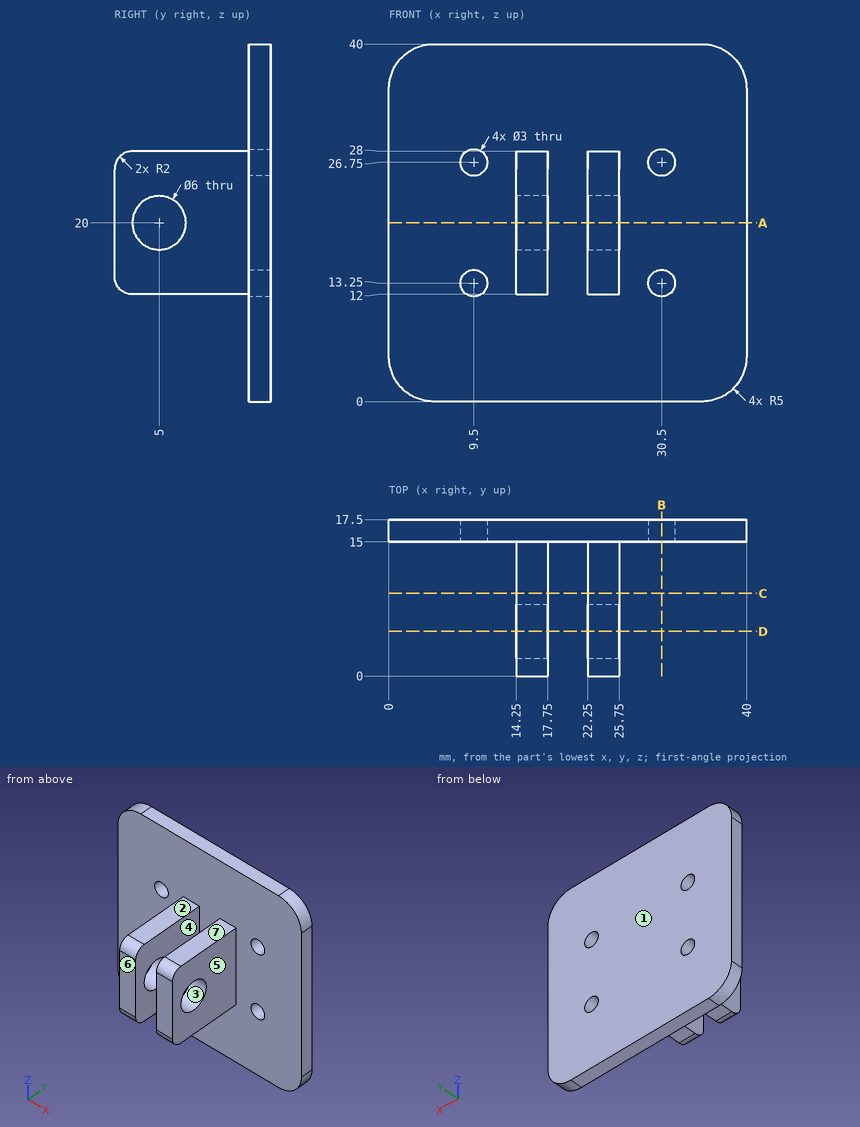
The drawing under review shows one solid part. Ordinate dimensions are in mm from its lowest x, y, z. A direction names the side the tool comes from. Coordinates: 2 decimals unless noted, no trailing zeros. Write each loop counter-clockwise with the first axis right and the second up, starting at its lowest first coordinate (ties: lowest second). Pieces come first, ordered by that corner, then holes.
1) Mouldability with a two-part tool opening along Y and no side actions: class the marked faces 1, 2 and 3 as +Y half, -Y half, draft (parallel to the pull), parting line (faces both ways), or undercut.
2) Add section D-D (y = 5). Write out the cut boundary in (x, z).
3) Add section B-B (x = 30.5). Write out the cut boundary in (y, z).
4) Add section C-C (y = 9.25). Write out the cut boundary in (x, z).
5) Machinability: for the marked faces 4, 5, 6 and 7, which of the approach directions +Z, -Z, +X, -X, +Y, -Y give a long, thin tool a straight path to every point of the face, cutting with its end or side? Answer none if there is none.
6) Add section A-A (z = 20). Write out the cut boundary in (x, y), plus the area to 3 significant figures.
7) To check wall thickness, follow L1, parallel to X at y = 16.25, z = 13.25; L2, parallel to X at y = 9, z = 17.5; L3, parallel to Y at x = 15, z = 20. State the ranges of each line that lie inside material, in increasing order.
8) Insertion check: pin 1 (2.5 mm diameter, centred on x = 9.5, z = 13.25, fed in from +Y); pin 2 (3 mm diameter, centred on y = 9, z = 17, fed in from +X); pin 3 (1.8 mm diameter, centred on x = 23.5, y = 9.5, fed in from +Z); pin 4 (12 mm diameter, centred on x = 13.5, z = 17, fed in from -Y). Each pin has a flat end and moves straight along its axis. Give the tip position at first contact, or say it passes through.
Check result:
1. face 1: +Y half
1. face 2: draft
1. face 3: undercut
2. outline: (14.25, 12) - (17.75, 12) - (17.75, 17) - (14.25, 17) - close; (14.25, 23) - (17.75, 23) - (17.75, 28) - (14.25, 28) - close; (22.25, 12) - (25.75, 12) - (25.75, 17) - (22.25, 17) - close; (22.25, 23) - (25.75, 23) - (25.75, 28) - (22.25, 28) - close
3. outline: (15, 0) - (17.5, 0) - (17.5, 11.75) - (15, 11.75) - close; (15, 14.75) - (17.5, 14.75) - (17.5, 25.25) - (15, 25.25) - close; (15, 28.25) - (17.5, 28.25) - (17.5, 40) - (15, 40) - close
4. outline: (14.25, 12) - (17.75, 12) - (17.75, 28) - (14.25, 28) - close; (22.25, 12) - (25.75, 12) - (25.75, 28) - (22.25, 28) - close
5. face 4: +Z, -Z, -Y
5. face 5: +Z, -Z, +X, -Y
5. face 6: +Z, -Z, +X, -X, -Y
5. face 7: +Z, +X, -X, -Y
6. outline: (0, 15) - (14.25, 15) - (14.25, 8) - (17.75, 8) - (17.75, 15) - (22.25, 15) - (22.25, 8) - (25.75, 8) - (25.75, 15) - (40, 15) - (40, 17.5) - (0, 17.5) - close; (14.25, 0) - (17.75, 0) - (17.75, 2) - (14.25, 2) - close; (22.25, 0) - (25.75, 0) - (25.75, 2) - (22.25, 2) - close
6. area: 163 mm2
7. L1: x = 0 to 8, 11 to 29, 32 to 40
7. L2: x = 14.25 to 17.75, 22.25 to 25.75
7. L3: y = 0 to 2, 8 to 17.5
8. pin 1: passes through
8. pin 2: stops at x = 25.75
8. pin 3: stops at z = 28
8. pin 4: stops at y = 0
